Can you work these out from the drawing? Everything is in mm from the part's minimum corner. A direction names the side the tool comes from. Coordinates: 2 decimals unless noted, no trailing zeros. Loops run counter-clockwise (first coordinate to the right, second up) from the corner with the lowest first, then second, coordinate; pieces in that order, holes last. Notation, with made-up numbers: (8, -25.75) - (42, -25.75) arc R28 cw to (42, 3.25) - close; hole circle Ø8 at (61.5, 4.5). An arc over 180 degrees is marked (long way). Use CSV: the item, a comma, the result in double quotes.
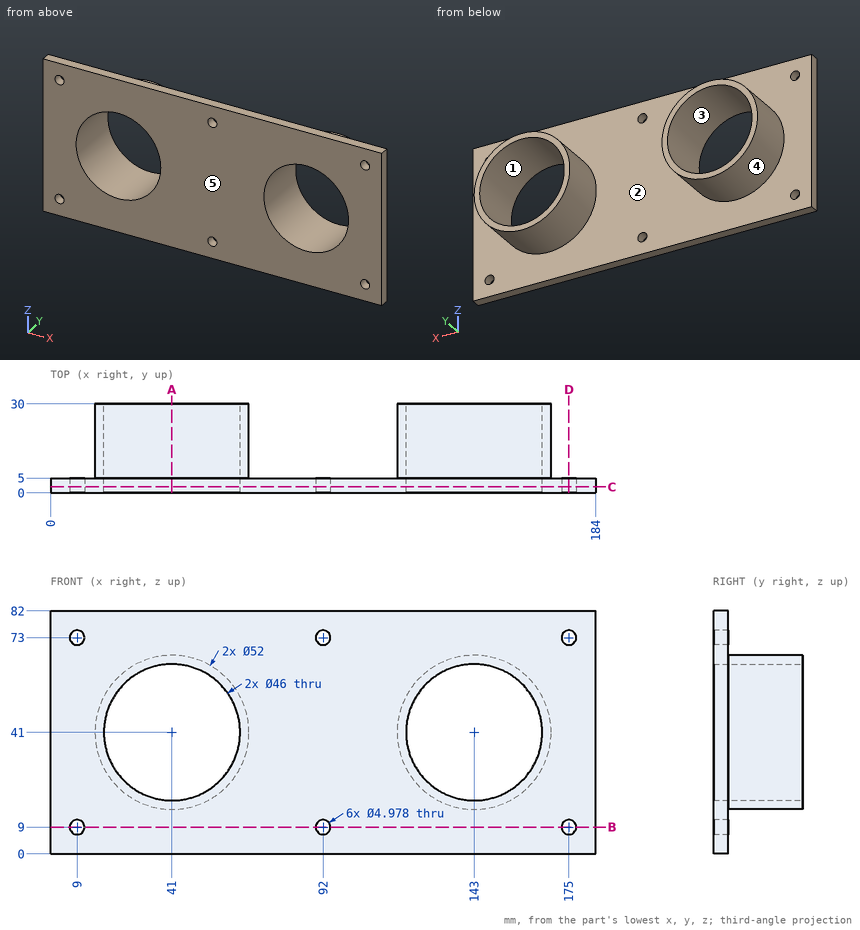
(1) Suppose I cut it at A-A (x = 41). Write out the boundary of the cut face in (y, z).
Computed:
outline,"(0, 0) - (5, 0) - (5, 15) - (30, 15) - (30, 18) - (0, 18) - close; (0, 64) - (30, 64) - (30, 67) - (5, 67) - (5, 82) - (0, 82) - close"
(2) Will these pins go through, and if not, where does the flat tip stop? pin 1 (8 mm diameter, centred on x = 92, z = 9, fed in from -Y); pin 2 (1 mm diameter, centred on x = 76, z = 61.5, fed in from +Y).
Computed:
pin 1,"stops at y = 0"
pin 2,"stops at y = 5"
(3) Please list where these lines run through material, in increasing order: line 1 (Z direction, x = 175, y = 2.45); line 2 (X direction, y = 3.55, z = 9); line 3 (X direction, y = 11.25, z = 29) (1 decimal).
Computed:
line 1,"z = 0 to 6.51, 11.49 to 70.51, 75.49 to 82"
line 2,"x = 0 to 6.51, 11.49 to 89.51, 94.49 to 172.51, 177.49 to 184"
line 3,"x = 17.9 to 21.4, 60.6 to 64.1, 119.9 to 123.4, 162.6 to 166.1"
(4) Suppose I cut it at C-C (y = 2). State how many separate pieces and enclosed holes the cut face has, plus the area to 3 significant figures.
Computed:
separate pieces,"1"
enclosed holes,"8"
area,"11,600 mm²"
(5) Suppose I cut it at B-B (z = 9). Write out the boundary of the cut face in (x, y).
Computed:
outline,"(0, 0) - (6.51, 0) - (6.51, 5) - (0, 5) - close; (11.49, 0) - (89.51, 0) - (89.51, 5) - (11.49, 5) - close; (94.49, 0) - (172.51, 0) - (172.51, 5) - (94.49, 5) - close; (177.49, 0) - (184, 0) - (184, 5) - (177.49, 5) - close"
(6) Which directions (+Z, -Z, +X, -X, +Y, -Y) give clear straight access to the entire face, cutting with the end or side of a thin tool? Please do the marked faces 1 and 2.
Computed:
face 1,"+Y, -Y"
face 2,"+Y"
(7) Suppose I cut it at D-D (x = 175). Write out the boundary of the cut face in (y, z), plus the area to 3 significant figures.
Computed:
outline,"(0, 0) - (5, 0) - (5, 6.51) - (0, 6.51) - close; (0, 11.49) - (5, 11.49) - (5, 70.51) - (0, 70.51) - close; (0, 75.49) - (5, 75.49) - (5, 82) - (0, 82) - close"
area,"360 mm²"
(8) Thinking about a two-plate mould opening in X: for the marked faces 3, 4 and 5, which applies, +X half, -X half, draft (parallel to the pull), parting line (faces both ways), or undercut?
Computed:
face 3,"undercut"
face 4,"undercut"
face 5,"draft"
